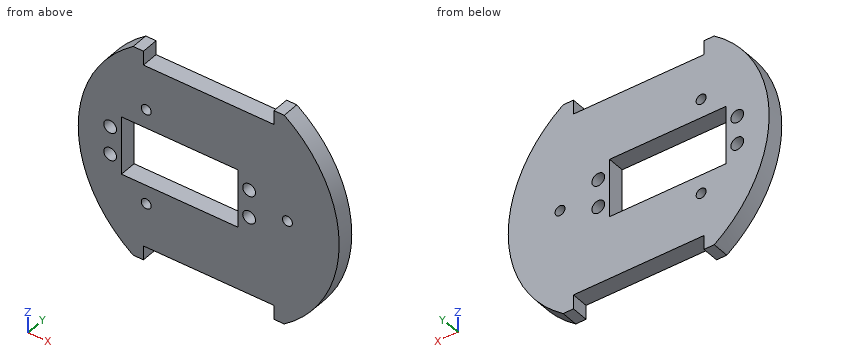
```python
from build123d import *

# Parameters (mm, degrees)
SKETCH1_R           = 2.25
SKETCH1_R_2         = 1.75
SKETCH1_W           = 41
SKETCH1_H           = 20.6
BOSS_EXTRUDE1_DEPTH = 6


with BuildPart() as part:
    # Sketch1 → Boss-Extrude1 (new body)
    with BuildSketch(Plane(origin=(0, 0, 0), x_dir=(1, 0, 0), z_dir=(0, 1, 0))):
        with BuildLine():
            Line((-26.64113361, 37.5), (-23, 37.5))
            Line((-23, 37.5), (-23, 32.5))
            Line((-23, 32.5), (23, 32.5))
            Line((23, 32.5), (23, 37.5))
            Line((23, 37.5), (26.64113361, 37.5))
            ThreePointArc((26.64113361, 37.5), (46, 0), (26.64113361, -37.5))
            Line((26.64113361, -37.5), (23, -37.5))
            Line((23, -37.5), (23, -32.5))
            Line((23, -32.5), (-23, -32.5))
            Line((-23, -32.5), (-23, -37.5))
            Line((-23, -37.5), (-26.64113361, -37.5))
            ThreePointArc((-26.64113361, -37.5), (-46, 0), (-26.64113361, 37.5))
        make_face()
        with Locations(Location((14.25, 4.9, 0), (0, 0, 270))):
            Circle(SKETCH1_R, mode=Mode.SUBTRACT)
        with Locations(Location((14.25, -4.9, 0), (0, 0, 270))):
            Circle(SKETCH1_R, mode=Mode.SUBTRACT)
        with Locations(Location((-34.75, 4.9, 0), (0, 0, 90))):
            Circle(SKETCH1_R, mode=Mode.SUBTRACT)
        with Locations(Location((-34.75, -4.9, 0), (0, 0, 90))):
            Circle(SKETCH1_R, mode=Mode.SUBTRACT)
        with Locations(Location((27.75, 0, 0), (0, 0, 270))):
            Circle(SKETCH1_R_2, mode=Mode.SUBTRACT)
        with Locations(Location((-22.015555193, 16.893129655, 0), (0, 0, 270))):
            Circle(SKETCH1_R_2, mode=Mode.SUBTRACT)
        with Locations(Location((-22.015555193, -16.893129655, 0), (0, 0, 270))):
            Circle(SKETCH1_R_2, mode=Mode.SUBTRACT)
        with Locations((-10.25, 0)):
            Rectangle(SKETCH1_W, SKETCH1_H, mode=Mode.SUBTRACT)
    extrude(amount=BOSS_EXTRUDE1_DEPTH)


solid = part.part
```
Design review of the part built by this model. Coordinates are the model's own, in mm. Coordinates: 2 decimals unless noted, no trailing zeros. Order: outer loops, then holes, each group sorted by start corner. A loop starts at its lowest first (then second) coordinate and runs counter-clockwise, first axis right, second up. Notation, with made-up numbers: (-16.75, 52.25) -> (13.25, 52.25) arc R20 cw to (13.25, 70.25) -> close; hole circle Ø3 at (8, 75.25). An arc over 180 degrees is marked (long way). One line per item, written item: value. Start each with the question number.
Q1. Take a section at A-A, the plane x = 14.25. State the section outline as (y, z) points, then the cut area to 3 significant figures.
Q2. For probe 1 along Z at (x, y) = (-22, 0.5); probe 2 along X at (y, z) = (2.5, -4.9); probe 3 along X at (y, z) = (4.95, -1), list the stretches that pass through material, from the lowest coordinate up.
Q3. Take a section at D-D, the plane y = 3.25. Give the number of separate pieces and of enclosed holes in the cut face, then the cut area to 3 significant figures.
Q4. Take a section at B-B, the plane z = 0. State the section outline as (x, y) points.
Q5. Take a section at C-C, the plane x = 27.75. State the section outline as (y, z) points, then the cut area to 3 significant figures.
Q6. Insertion check: pin 1 Ø2 at (x, y) = (-6, 1.5) entering from +Z; pin 2 Ø12 at (x, z) = (20, 6) entering from -Y; pin 3 Ø2.5 at (y, z) = (2, -34) entering from +X; pin 4 Ø1.8 at (y, z) = (2, 2.5) entering from -X. Each pin has a flat end and moves straight along its axis. Give the tip position at first contact, or say it passes through.
Values follow:
1. outline: (0, -32.5) -> (6, -32.5) -> (6, -7.15) -> (0, -7.15) -> close; (0, -2.65) -> (6, -2.65) -> (6, 2.65) -> (0, 2.65) -> close; (0, 7.15) -> (6, 7.15) -> (6, 32.5) -> (0, 32.5) -> close
1. area: 336 mm2
2. probe 1: z = -32.5 to -18.64, -15.14 to -10.3, 10.3 to 15.14, 18.64 to 32.5
2. probe 2: x = -45.74 to -37, -32.5 to -30.75, 10.25 to 12, 16.5 to 45.74
2. probe 3: x = -45.99 to -30.75, 10.25 to 26.31, 29.19 to 45.99
3. separate pieces: 1
3. enclosed holes: 8
3. area: 4,630 mm2
4. outline: (-46, 0) -> (-30.75, 0) -> (-30.75, 6) -> (-46, 6) -> close; (10.25, 0) -> (26, 0) -> (26, 6) -> (10.25, 6) -> close; (29.5, 0) -> (46, 0) -> (46, 6) -> (29.5, 6) -> close
5. outline: (0, -36.69) -> (6, -36.69) -> (6, -1.75) -> (0, -1.75) -> close; (0, 1.75) -> (6, 1.75) -> (6, 36.69) -> (0, 36.69) -> close
5. area: 419 mm2
6. pin 1: stops at z = 32.5
6. pin 2: stops at y = 0
6. pin 3: stops at x = 32.3
6. pin 4: stops at x = -45.97
